```python
from build123d import *

# Parameters (mm, degrees)
F0_R     = 8
F0_R_2   = 4
F1_DEPTH = 2
F2_DEPTH = 10
F3_SIZE  = 0.2


with BuildPart() as f1:
    # F0 (on Top) → F1 (new body)
    with BuildSketch(Plane.XY):
        Circle(F0_R)
        with BuildLine():
            ThreePointArc((-3.3166247904, -5), (-6, 0), (-3.3166247904, 5))
            Line((-3.3166247904, 5), (3.3166247904, 5))
            ThreePointArc((3.3166247904, 5), (6, 0), (3.3166247904, -5))
            Line((3.3166247904, -5), (-3.3166247904, -5))
        make_face(mode=Mode.SUBTRACT)
        with BuildLine():
            Line((3.3166247904, 5), (-3.3166247904, 5))
            ThreePointArc((-3.3166247904, 5), (-6, 0), (-3.3166247904, -5))
            Line((-3.3166247904, -5), (3.3166247904, -5))
            ThreePointArc((3.3166247904, -5), (6, 0), (3.3166247904, 5))
        make_face()
        Circle(F0_R_2, mode=Mode.SUBTRACT)
    extrude(amount=F1_DEPTH)

    # F0 (on Top) → F2 (join)
    with BuildSketch(Plane.XY):
        with BuildLine():
            Line((3.3166247904, 5), (-3.3166247904, 5))
            ThreePointArc((-3.3166247904, 5), (-6, 0), (-3.3166247904, -5))
            Line((-3.3166247904, -5), (3.3166247904, -5))
            ThreePointArc((3.3166247904, -5), (6, 0), (3.3166247904, 5))
        make_face()
        Circle(F0_R_2, mode=Mode.SUBTRACT)
    extrude(amount=-F2_DEPTH)

    # F3
    f3_edges = [f1.edges().sort_by_distance(p)[0] for p in [
        (-8, 0, 2),
        (-6, 0, -10),
        (0, 5, -10),
        (6, 0, -10),
        (0, -5, -10),
    ]]
    chamfer(f3_edges, length=F3_SIZE)


solid = f1.part
```
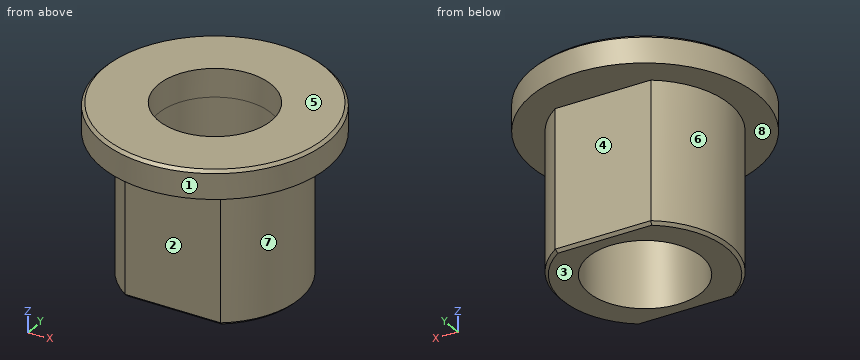
CAD build for the part. Positions are in the model's coordinates, mm. Face numbers are marked on the shaded views. A direction names the side the tool comes from. Give positions to 0.01 mm unless a question says otherwise; leave off trailing zeros. Loops run counter-clockwise (first coordinate to the right, second up) from the corner with the lowest first, then second, coordinate; pieces in that order, holes last. Notation, with made-up numbers: (-36.5, 81) - (2.5, 81) arc R22 cw to (2.5, 95) - close; hole circle Ø5 at (60, -36). An arc over 180 degrees is marked (long way). Put each result on its own line as item: value.
Q1. Mould opens along Y. For the marked faces 1, 2, 3 and 4 say: pulls with the +Y half, pulls with the -Y half, needs draft (parallel to the pull), parting line crosses it, or undercut.
Filled in:
face 1: parting line crosses it
face 2: pulls with the -Y half
face 3: needs draft
face 4: pulls with the +Y half
Q2. Probe line 1 along Y through (x, z) = (0, -6); line 2 along Z through (x, y) = (-7, -1.25); line 3 along Y through (x, z) = (0.25, 1.5). List the from-to ranges inside material, lowest first.
Filled in:
line 1: y = -5 to -4, 4 to 5
line 2: z = 0 to 2
line 3: y = -8 to -3.99, 3.99 to 8
Q3. Tool access for the marked faces 5, 6, 7 and 8: list every direction of +Z, -Z, +X, -X, +Y, -Y with a clear straight run to the whole face (end or side of a thin tool).
Filled in:
face 5: +Z, +X, -X, +Y, -Y
face 6: -Z, -X
face 7: -Z, +X
face 8: -Z
Q4. Flat gauge pin, fed straight in: pin 1 (2 mm diameter, centred on x = 1, z = -4, fed in from +Y). Where does the tip first touch, or does it go through?
Filled in:
pin 1: stops at y = 5
Q5. Slice it at B-B (x = 0). Give the cut face in (y, z).
Filled in:
outline: (-8, 0) - (-5, 0) - (-5, -9.8) - (-4.8, -10) - (-4, -10) - (-4, 2) - (-7.8, 2) - (-8, 1.8) - close; (4, -10) - (4.8, -10) - (5, -9.8) - (5, 0) - (8, 0) - (8, 1.8) - (7.8, 2) - (4, 2) - close
Q6. Slice it at C-C (z = -4). Give the cut face in (x, y).
Filled in:
outline: (-3.32, -5) - (3.32, -5) arc R6 ccw to (3.32, 5) - (-3.32, 5) arc R6 ccw to start; hole circle Ø8 at (0, 0)
Q7. Slice it at A-A (y = 0). Give the cut face in (x, z), plus the area to 3 significant figures.
Filled in:
outline: (-8, 0) - (-6, 0) - (-6, -9.8) - (-5.8, -10) - (-4, -10) - (-4, 2) - (-7.8, 2) - (-8, 1.8) - close; (4, -10) - (5.8, -10) - (6, -9.8) - (6, 0) - (8, 0) - (8, 1.8) - (7.8, 2) - (4, 2) - close
area: 55.9 mm²
